Read the model definition and answer for the solid it produces. Units are mm, in the model's axes. Coordinates: 2 decimals unless noted, no trailing zeros. Write each loop counter-clockwise with the first axis right and the second up, starting at its lowest first coordinate (ties: lowest second). Pieces come first, ordered by that corner, then holes. Notation, with made-up numbers: (-11, -32.75) -> (32, -32.75) arc R34 ccw to (32, -2.75) -> close; hole circle Ø5 at (-10.75, 82.5). An arc over 180 degrees is marked (long way). Write item = value, one per line. Start each with the question number.
1) Find the intervals of material crossed by line 1 along X through (y, z) = (127, 26.35); line 2 along X through (y, z) = (100.5, 26.95); line 3 along Y through (x, z) = (-101, 27.15), in increasing order. Write a range as from..to.
2) Section B-B (z = 27.8) is taken. Count the separate pieces of the cut face and the enclosed holes in it, plus the area to 3 significant figures.
3) Flat-ended cylindrical pins translate along their axes: pin 1 Ø4 at (x, y) = (-152.8, 73.5) entering from +Z; pin 2 Ø5.5 at (x, y) = (-49, 46.75) entering from +Z; pin 3 Ø4.5 at (x, y) = (-152.8, 127) entering from +Z. Find the tip coordinate at first contact, or state that the pin passes through.
4) Section A-A (x = -97) is taken. Determine the outline of the cut face in (y, z), plus the area to 3 significant figures.
from build123d import *

# Parameters (mm, degrees)
SKETCH068_W         = 112.8
SKETCH068_H         = 130
PAD003_DEPTH        = 3
HOLE015_D           = 3.3
HOLE015_DEPTH       = 3
HOLE015_CSINK_D     = 5.6
HOLE015_CSINK_ANGLE = 90
SKETCH073_W         = 10.6
SKETCH073_H         = 5.6
POCKET016_DEPTH     = 5
FILLET001_R         = 3.35


with BuildPart() as part:
    # Sketch068 → Pad003 (new body)
    with BuildSketch(Plane.XY):
        with Locations((-100.900002, 75)):
            Rectangle(SKETCH068_W, SKETCH068_H)
    extrude(amount=PAD003_DEPTH)

    # Hole015
    with Locations(Plane.XY.offset(3)):
        with Locations((-152.800002, 20.000492), (-152.800002, 46.749416), (-152.800002, 73.500001), (-152.800002, 100.249657), (-152.800002, 126.999153), (-49.000002, 20.001339), (-49.000002, 46.750263), (-49.000002, 73.500848), (-49.000002, 100.250504), (-49.000002, 127)):
            CounterSinkHole(HOLE015_D / 2, HOLE015_CSINK_D / 2, depth=HOLE015_DEPTH, counter_sink_angle=HOLE015_CSINK_ANGLE)

    # Sketch073 (on Face5 of Hole015) → Pocket016 (cut)
    with BuildSketch(Plane.XY.offset(3)):
        with Locations((-100.839996, 15.79)):
            Rectangle(SKETCH073_W, SKETCH073_H)
    extrude(amount=-POCKET016_DEPTH, mode=Mode.SUBTRACT)

    # Fillet001
    fillet001_edges = [part.edges().sort_by_distance(p)[0] for p in [
        (-44.500002, 140, 1.5),
        (-157.300002, 140, 1.5),
    ]]
    fillet(fillet001_edges, radius=FILLET001_R)


with BuildPart() as part_1:
    # Body009 placement: moved
    add(part.part.moved(Location((0, 0, 25.3))))


solid = part_1.part
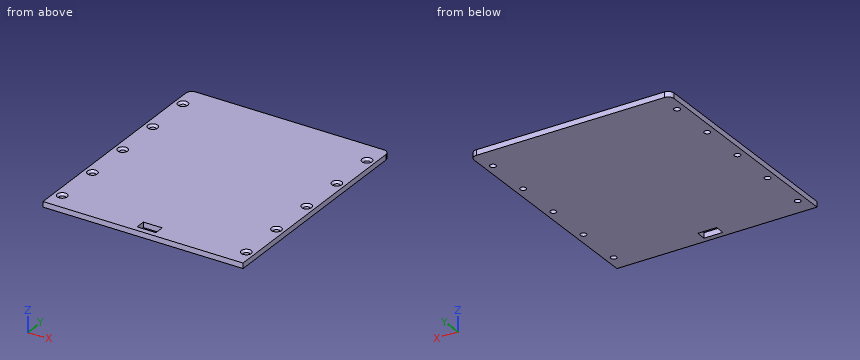
Answer key:
q1.line_1 = -157.3..-154.45, -151.15..-50.65, -47.35..-44.5
q1.line_2 = -157.3..-154.43, -151.17..-50.63, -47.37..-44.5
q1.line_3 = 10..12.99, 18.59..140
q2.separate_pieces = 1
q2.enclosed_holes = 11
q2.area = 14,400 mm^2
q3.pin_1 = 27.5
q3.pin_2 = 28.25
q3.pin_3 = 27.75
q4.outline = (10, 25.3) -> (12.99, 25.3) -> (12.99, 28.3) -> (10, 28.3) -> close; (18.59, 25.3) -> (140, 25.3) -> (140, 28.3) -> (18.59, 28.3) -> close
q4.area = 373 mm^2
